Autodesk Inventor part; units mm, degrees
ref_plane "YZ Plane" through (0, 0, 0) normal (1, 0, 0) x (0, 1, 0)
ref_plane "XZ Plane" through (0, 0, 0) normal (0, 1, 0) x (-1, 0, 0)
ref_plane "XY Plane" through (0, 0, 0) normal (0, 0, 1) x (1, 0, 0)
sketch "Náčrt1" plane through (0, 0, 0) normal (0, 1, 0) x (-1, 0, 0)
  line L0 (0, -93.1) -> (0, 93.1)
  line L1 (-121.1, 0) -> (121.1, 0)
  line L2 (86.5, 66.5) -> (-86.5, 66.5)
  line L3 (-86.5, 66.5) -> (-86.5, -66.5)
  line L4 (-86.5, -66.5) -> (86.5, -66.5)
  line L5 (86.5, -66.5) -> (86.5, 66.5)
  point P0 (0, 0)
  dimension "d0" = 133
  dimension "d1" = 173
extrude "Vysunutí1" add sketch "Náčrt1" along normal mid plane 3
sketch "Náčrt2" plane through (0, 1.5, 0) normal (0, 1, 0) x (1, 0, 0)
  line L0 (-61.5, -46.5) -> (-11.5, -46.5)
  line L1 (-11.5, -46.5) -> (-11.5, 3.5)
  line L2 (-11.5, 3.5) -> (-61.5, 3.5)
  line L3 (-61.5, 3.5) -> (-61.5, -46.5)
  line L4 (-86.5, -66.5) -> (86.5, -66.5)
  line L5 (-86.5, 66.5) -> (-86.5, -66.5)
  point P0 (0, 0)
  dimension "d4" = 50
  dimension "d5" = 50
  dimension "d12" = 25
  dimension "d13" = 20
extrude "Vysunutí3" cut sketch "Náčrt2" against normal through all
sketch "Náčrt3" plane through (0, 1.5, 0) normal (0, 1, 0) x (1, 0, 0)
  line L0 (-86.5, -66.5) -> (86.5, -66.5)
  line L1 (86.5, -66.5) -> (86.5, 66.5)
  point P0 (0, 0)
  point P1 (66.5, -41.5)
  dimension "d19" = 20
  dimension "d20" = 25
hole "Díra1" at (66.5, 1.5, 41.5) direction (0, -1, 0) diameter 20 end through all
properties part number "Cabinet - left"
Input: part model. Units: mm. Frame: model coordinates. Round coordinates to 2 decimals unless told otherwise and drop trailing zeros. Order: outer loops, then holes, each group sorted by start corner. A loop starts at its lowest first (then second) coordinate and runs counter-clockwise, first axis right, second up.
1. Cut plane C-C, the plane z = 5.5. Output: boundary loops of the cut face in (x, y), then the cut area to 3 significant figures.
The answers:
outline: (-86.5, -1.5) - (-61.5, -1.5) - (-61.5, 1.5) - (-86.5, 1.5) - close; (-11.5, -1.5) - (86.5, -1.5) - (86.5, 1.5) - (-11.5, 1.5) - close
area: 369 mm2
2. Cut plane B-B, the plane z = 41.5. Output: boundary loops of the cut face in (x, y), then the cut area to 3 significant figures.
The answers:
outline: (-86.5, -1.5) - (-61.5, -1.5) - (-61.5, 1.5) - (-86.5, 1.5) - close; (-11.5, -1.5) - (56.5, -1.5) - (56.5, 1.5) - (-11.5, 1.5) - close; (76.5, -1.5) - (86.5, -1.5) - (86.5, 1.5) - (76.5, 1.5) - close
area: 309 mm2
3. Cut plane D-D, the plane y = 0.4. Output: boundary loops of the cut face in (x, z).
The answers:
outline: (-86.5, -66.5) - (86.5, -66.5) - (86.5, 66.5) - (-86.5, 66.5) - close; hole (-61.5, -3.5) - (-11.5, -3.5) - (-11.5, 46.5) - (-61.5, 46.5) - close; hole circle Ø20 at (66.5, 41.5)
4. Material intervals for line 1 (X direction, y = -0.1, z = 41.5); line 2 (X direction, y = -0.7, z = 1); line 3 (Z direction, x = 66.5, y = -0.35), sorted ascending.
The answers:
line 1: x = -86.5 to -61.5, -11.5 to 56.5, 76.5 to 86.5
line 2: x = -86.5 to -61.5, -11.5 to 86.5
line 3: z = -66.5 to 31.5, 51.5 to 66.5
5. Cut plane A-A, the plane x = 66.5. Output: boundary loops of the cut face in (y, z), then the cut area to 3 significant figures.
The answers:
outline: (-1.5, -66.5) - (1.5, -66.5) - (1.5, 31.5) - (-1.5, 31.5) - close; (-1.5, 51.5) - (1.5, 51.5) - (1.5, 66.5) - (-1.5, 66.5) - close
area: 339 mm2
6. Mould query, pull axis Z, two halves, no side actions, for faces 1 (the face through (76.26, -0.02, 39.33)), 2 (the face through (1, 1.5, 1)). Classes: released by +Z, released by -Z, zero draft, split by the parting line, or undercut.
The answers:
face 1: undercut
face 2: zero draft
